from build123d import *

# Parameters (mm, degrees)
SKETCH1_R           = 30
SKETCH1_R_2         = 20
BOSS_EXTRUDE1_DEPTH = 15
FILLET1_R           = 3
FILLET2_R           = 1.5


with BuildPart() as part:
    # Sketch1 → Boss-Extrude1 (new body)
    with BuildSketch(Plane(origin=(0, 0, 0), x_dir=(1, 0, 0), z_dir=(0, 1, 0))):
        Circle(SKETCH1_R)
        Circle(SKETCH1_R_2, mode=Mode.SUBTRACT)
    extrude(amount=BOSS_EXTRUDE1_DEPTH)

    # Fillet1
    fillet1_edges = [part.edges().sort_by_distance(p)[0] for p in [
        (-30, 0, 0),
        (-30, 15, 0),
    ]]
    fillet(fillet1_edges, radius=FILLET1_R)

    # Fillet2
    fillet2_edges = [part.edges().sort_by_distance(p)[0] for p in [
        (-20, 0, 0),
        (-20, 15, 0),
    ]]
    fillet(fillet2_edges, radius=FILLET2_R)


solid = part.part
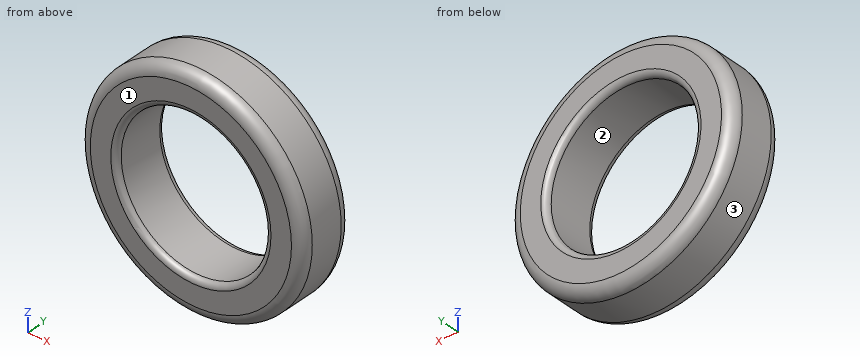
Verification items for the finished model (mm, model axes). Face numbers are marked on the shaded views. Round coordinates to 2 decimals unless told otherwise and drop trailing zeros. Loops run counter-clockwise (first coordinate to the right, second up) from the corner with the lowest first, then second, coordinate; pieces in that order, holes last. Notation, with made-up numbers: (82, 84.25) - (113, 84.25) arc R4 cw to (113, 90.25) - close; hole circle Ø3 at (-24, -10.75). An arc over 180 degrees is marked (long way). Answer in a Markdown table with one row per item. Add a question column.
Q1. Release check for a two-part mould opening along Z. For the marked faces 1, 2 and 3 record: pulls with the +Z half, pulls with the -Z half, needs draft (parallel to the pull), parting line crosses it, or undercut.
Q2. Section check A-A on z = 0. Enter the section's corners in (x, y), plus the area to 3 significant figures.
Q3. Section check B-B on x = 0. Enter the section's corners in (y, z), plus the area to 3 significant figures.
Q4. Gauge pin test, flat ends, axial feed: pin 1 (3 mm diameter, centred on x = -21.5, y = 6, fed in from -Z); pin 2 (1 mm diameter, centred on x = 24, y = 4.5, fed in from -Z); pin 3 (3 mm diameter, centred on x = 11, y = 12, fed in from -Z); pin 4 (1 mm diameter, centred on x = 17.5, z = 19, fed in from -Y). Record the tip position at first contact, or that the pin passes through.
Q5. Material ranges on line 1 (X direction, y = 8.75, z = 0); line 2 (X direction, y = 12.5, z = -17), recorded low to high.
Q6. Section check C-C on y = 8. Enter the section's corners in (x, z).
Found:
| question | item | result |
|---|---|---|
| 1 | face 1 | needs draft |
| 1 | face 2 | undercut |
| 1 | face 3 | parting line crosses it |
| 2 | outline | (-30, 3) arc R3 ccw to (-27, 0) - (-21.5, 0) arc R1.5 ccw to (-20, 1.5) - (-20, 13.5) arc R1.5 ccw to (-21.5, 15) - (-27, 15) arc R3 ccw to (-30, 12) - close; (20, 1.5) arc R1.5 ccw to (21.5, 0) - (27, 0) arc R3 ccw to (30, 3) - (30, 12) arc R3 ccw to (27, 15) - (21.5, 15) arc R1.5 ccw to (20, 13.5) - close |
| 2 | area | 290 mm² |
| 3 | outline | (0, -27) arc R3 ccw to (3, -30) - (12, -30) arc R3 ccw to (15, -27) - (15, -21.5) arc R1.5 ccw to (13.5, -20) - (1.5, -20) arc R1.5 ccw to (0, -21.5) - close; (0, 21.5) arc R1.5 ccw to (1.5, 20) - (13.5, 20) arc R1.5 ccw to (15, 21.5) - (15, 27) arc R3 ccw to (12, 30) - (3, 30) arc R3 ccw to (0, 27) - close |
| 3 | area | 290 mm² |
| 4 | pin 1 | stops at z = -22.36 |
| 4 | pin 2 | stops at z = -18.65 |
| 4 | pin 3 | stops at z = -28.46 |
| 4 | pin 4 | stops at y = 0 |
| 5 | line 1 | x = -30 to -20, 20 to 30 |
| 5 | line 2 | x = -24.67 to -10.54, 10.54 to 24.67 |
| 6 | outline | circle Ø60 at (0, 0); hole circle Ø40 at (0, 0) |
